Part model, mm, in its own coordinate system. Face numbers are marked on the shaded views. Round coordinates to 2 decimals unless told otherwise and drop trailing zeros. Write each loop counter-clockwise with the first axis right and the second up, starting at its lowest first coordinate (ties: lowest second). Pieces come first, ordered by that corner, then holes. Notation, with made-up numbers: M -1.5,34 L 12.5,34 A37 ccw 12.5,73 Z; hole C 87,35 d3. An arc over 180 degrees is marked long. One line per question, with ' | ' between items. Start each with the question number.
1) Drop flat-ended pins along their axis: pin 1 Ø1 at (y, z) = (3, -1) entering from -X; pin 2 Ø1.5 at (x, z) = (-0.5, 0.5) entering from +Y. Give the stop position or say it passes through.
2) Saw through at C-C (z = 0). List the corners of the cut face in (x, y), plus the area to 3 significant figures.
3) Mould opens along Y. For the marked faces 1, 2 and 3 say: pulls with the +Y half, pulls with the -Y half, needs draft (parallel to the pull), parting line crosses it, or undercut.
4) Saw through at D-D (y = 2). List the corners of the cut face in (x, z), plus the area to 3 significant figures.
5) Wall check: probe 1 along X at (y, z) = (6, 0); probe 2 along Y at (x, z) = (0.5, -0.75); probe 3 along Z at (x, y) = (0.25, 6). Give the ranges that are in metal, low to high. Write a range as [from, to].
6) Saw through at A-A (x = 0). List the corners of the cut face in (y, z), plus the area to 3 significant figures.
7) Saw through at B-B (y = 6.25). List the corners of the cut face in (x, z).
```python
from build123d import *

# Parameters (mm, degrees)
SCHIZZO1_R                   = 3.1
ESTRUSIONE_ESTRUSIONE1_DEPTH = 4
SCHIZZO1_3_R                 = 3
ESTRUSIONE_ESTRUSIONE2_DEPTH = 5
ESTRUSIONE_ESTRUSIONE3_START = 5
SCHIZZO1_4_R                 = 3.1
SCHIZZO1_4_R_2               = 1.5
ESTRUSIONE_ESTRUSIONE3_DEPTH = 3


with BuildPart() as part:
    # Schizzo1 → Estrusione-Estrusione1 (new body)
    with BuildSketch(Plane(origin=(0, 0, 0), x_dir=(1, 0, 0), z_dir=(0, 1, 0))):
        with Locations(Location((0, 0, 0), (0, 0, 270))):
            Circle(SCHIZZO1_R)
    extrude(amount=ESTRUSIONE_ESTRUSIONE1_DEPTH)

    # Schizzo1<3> → Estrusione-Estrusione2 (add)
    with BuildSketch(Plane(origin=(0, 0, 0), x_dir=(1, 0, 0), z_dir=(0, 1, 0))):
        with Locations(Location((0, 0, 0), (0, 0, 270))):
            Circle(SCHIZZO1_3_R)
    extrude(amount=ESTRUSIONE_ESTRUSIONE2_DEPTH)

    # Schizzo1<4> → Estrusione-Estrusione3 (add)
    with BuildSketch(Plane(origin=(0, 0, 0), x_dir=(1, 0, 0), z_dir=(0, 1, 0)).offset(ESTRUSIONE_ESTRUSIONE3_START)):
        with Locations(Location((0, 0, 0), (0, 0, 270))):
            Circle(SCHIZZO1_4_R)
        with Locations(Location((0, 0, 0), (0, 0, 270))):
            Circle(SCHIZZO1_4_R_2, mode=Mode.SUBTRACT)
    extrude(amount=ESTRUSIONE_ESTRUSIONE3_DEPTH)


solid = part.part
```
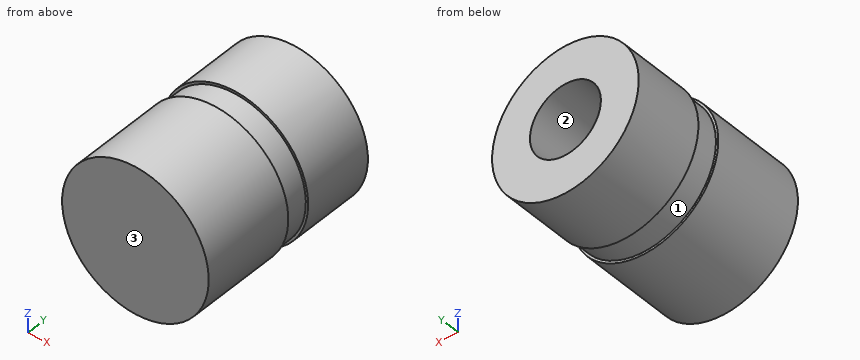
Answer key:
1) pin 1: stops at x = -3.06 | pin 2: stops at y = 5
2) outline: M -3.1,0 L 3.1,0 L 3.1,4 L 3,4 L 3,5 L 3.1,5 L 3.1,8 L 1.5,8 L 1.5,5 L -1.5,5 L -1.5,8 L -3.1,8 L -3.1,5 L -3,5 L -3,4 L -3.1,4 Z | area: 40.4 mm2
3) face 1: undercut | face 2: needs draft | face 3: pulls with the -Y half
4) outline: C 0,0 d6.2 | area: 30.2 mm2
5) probe 1: x = [-3.1, -1.5], [1.5, 3.1] | probe 2: y = [0, 5] | probe 3: z = [-3.09, -1.48], [1.48, 3.09]
6) outline: M 0,-3.1 L 4,-3.1 L 4,-3 L 5,-3 L 5,-3.1 L 8,-3.1 L 8,-1.5 L 5,-1.5 L 5,1.5 L 8,1.5 L 8,3.1 L 5,3.1 L 5,3 L 4,3 L 4,3.1 L 0,3.1 Z | area: 40.4 mm2
7) outline: C 0,0 d6.2; hole C 0,0 d3
